The model under review builds one solid part; all positions refer to its coordinate system, in mm. Face numbers are marked on the shaded views. A direction names the side the tool comes from. Give positions to 0.01 mm unless a question says otherwise; leave off trailing zeros. Write each loop counter-clockwise with the first axis right and the second up, starting at its lowest first coordinate (ties: lowest second). Pieces come first, ordered by that corner, then holes. Notation, with made-up numbers: (74, -38.5) - (95, -38.5) arc R17 ccw to (95, -29.5) - close; hole circle Ø11 at (28, 4). An arc over 180 degrees is marked (long way). Write item = value, one per line.
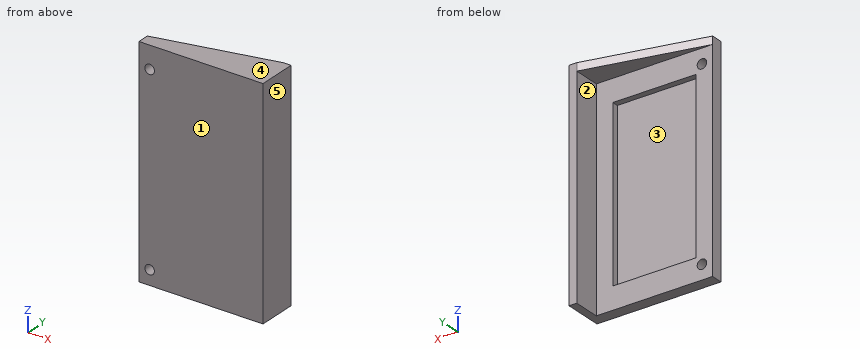
Autodesk Inventor part; units mm, degrees
ref_plane "YZ Plane" through (0, 0, 0) normal (1, 0, 0) x (0, 1, 0)
ref_plane "XZ Plane" through (0, 0, 0) normal (0, 1, 0) x (-1, 0, 0)
ref_plane "XY Plane" through (0, 0, 0) normal (0, 0, 1) x (1, 0, 0)
sketch "Sketch1" plane through (0, 0, 0) normal (0, 1, 0) x (-1, 0, 0)
  line L0 (-15, -27.5) -> (15, -27.5)
  line L1 (15, -27.5) -> (15, 27.5)
  line L2 (15, 27.5) -> (-15, 27.5)
  line L3 (-15, 27.5) -> (-15, -27.5)
  line L4 (-15, -27.5) -> (15, 27.5) construction
  line L5 (15, -27.5) -> (-15, 27.5) construction
  point P0 (0, 0)
  dimension "d0" = 55
  dimension "d1" = 30
extrude "Extrusion1" add sketch "Sketch1" along normal blind 3
sketch "Sketch2" plane through (0, 3, 0) normal (0, 1, 0) x (1, 0, 0)
  line L0 (10.75, 21.75) -> (-10.75, 21.75)
  line L1 (-10.75, 21.75) -> (-10.75, -21.75)
  line L2 (-10.75, -21.75) -> (10.75, -21.75)
  line L3 (10.75, -21.75) -> (10.75, 21.75)
  line L4 (10.75, 21.75) -> (-10.75, -21.75) construction
  line L5 (-10.75, 21.75) -> (10.75, -21.75) construction
  point P0 (0, 0)
  dimension "d4" = 43.5
  dimension "d5" = 21.5
extrude "Extrusion2" cut sketch "Sketch2" against normal blind 1.6
sketch "Sketch3" plane through (15, 0, 27.5) normal (1, 0, 0) x (0, 0, -1)
  line L0 (55, 0) -> (0, 0)
  line L1 (0, 0) -> (55, 0)
  line L2 (55, 0) -> (55, 10)
  line L3 (55, 10) -> (0, 10)
  line L4 (0, 10) -> (0, 0)
  line L5 (55, 0) -> (55, 3)
  point P0 (27.5, 0)
  dimension "d8" = 10
extrude "Extrusion3" add sketch "Sketch3" along normal blind 2
sketch "Sketch4" plane through (-15, 0, 27.5) normal (0, 0, 1) x (1, 0, 0)
  line L0 (0, 0) -> (32, 0)
  line L1 (32, 10) -> (32, 0)
  line L2 (30, 10) -> (32, 10)
  line L3 (30, 10) -> (30, 3)
  line L4 (0, 3) -> (30, 3)
  line L5 (0, 0) -> (0, 3)
  line L6 (0, 3) -> (30, 3)
  line L7 (30, 10) -> (32, 10)
  line L8 (0, 3) -> (30, 10)
  point P0 (15, 0)
extrude "Extrusion4" add sketch "Sketch4" along normal blind 2
sketch "Sketch5" plane through (0, 3, 0) normal (0, 1, 0) x (1, 0, 0)
  line L0 (12.25, 23.75) -> (-12.25, 23.75)
  line L1 (-12.25, 23.75) -> (-12.25, -23.75)
  line L2 (-12.25, -23.75) -> (12.25, -23.75)
  line L3 (12.25, -23.75) -> (12.25, 23.75)
  line L4 (12.25, 23.75) -> (-12.25, -23.75) construction
  line L5 (-12.25, 23.75) -> (12.25, -23.75) construction
  line L6 (-10.75, -21.75) -> (-10.75, 21.75)
  line L7 (10.75, -21.75) -> (-10.75, -21.75)
  point P0 (0, 0)
  dimension "d13" = 1.5
  dimension "d14" = 2
hole "Hole1" at (-12.25, 3, 23.75) at (-12.25, 3, -23.75) direction (0, -1, 0) diameter 2.459 end through all
properties part number "Buck_Bracket"
1. For line 1 (Z direction, x = -12.25, y = 2.1); line 2 (X direction, y = 1.5, z = 10); line 3 (X direction, y = 1.15, z = -23.75), list the stretches that pass through material, from the lowest coordinate up. Write a range as from..to.
Findings below:
line_1 = -27.5..-24.98, -22.52..22.52, 24.98..29.5
line_2 = -15..-10.75, 10.75..17
line_3 = -15..-13.48, -11.02..17
2. Take a section at A-A on z = -23.75. Give the boundary of the cut face in (x, y), and give its area (3 significant figures).
Findings below:
outline = (-15, 0) - (-13.48, 0) - (-13.48, 3) - (-15, 3) - close; (-11.02, 0) - (17, 0) - (17, 10) - (15, 10) - (15, 3) - (-11.02, 3) - close
area = 103 mm²
3. Machinability: for the marked faces 1 and 2, which of the approach directions +Z, -Z, +X, -X, +Y, -Y give a long, thin tool a straight path to every point of the face, cutting with its end or side? Answer none if there is none.
Findings below:
face_1 = +Z, -Z, +X, -X, -Y
face_2 = -Z, -X, +Y
4. Take a section at D-D on x = -3. Give the boundary of the cut face in (y, z).
Findings below:
outline = (0, -27.5) - (3, -27.5) - (3, -21.75) - (1.4, -21.75) - (1.4, 21.75) - (3, 21.75) - (3, 27.5) - (5.8, 27.5) - (5.8, 29.5) - (0, 29.5) - close
5. Take a section at B-B on x = -12.25. Give the boundary of the cut face in (y, z), and give its area (3 significant figures).
Findings below:
outline = (0, -27.5) - (3, -27.5) - (3, -24.98) - (0, -24.98) - close; (0, -22.52) - (3, -22.52) - (3, 22.52) - (0, 22.52) - close; (0, 24.98) - (3, 24.98) - (3, 27.5) - (3.64, 27.5) - (3.64, 29.5) - (0, 29.5) - close
area = 158 mm²
6. Take a section at C-C on z = 3. Give the boundary of the cut face in (x, y).
Findings below:
outline = (-15, 0) - (17, 0) - (17, 10) - (15, 10) - (15, 3) - (10.75, 3) - (10.75, 1.4) - (-10.75, 1.4) - (-10.75, 3) - (-15, 3) - close
7. Draft analysis for pull direction X (two halves, no side actions). For the marked faces 3, 4 and 5, state which applies: +X half, -X half, draft (parallel to the pull), parting line (faces both ways), or undercut.
Findings below:
face_3 = undercut
face_4 = draft
face_5 = +X half
8. Insertion check: P1, Ø1.5, axis at x = -12.25, z = 23.75, coming from the -Y side; P2, Ø1, axis at x = 10.5, y = 8.5, coming from the -Z side; P3, Ø5, axis at x = -11.5, z = -11, coming from the +Y side; P4, Ø2, axis at y = 8, z = 12, coming from the -X side. Each pin has a flat end and moves straight along its axis. Give the tip position at first contact, or say it passes through.
Findings below:
P1 = through
P2 = 27.5
P3 = 3
P4 = 15
